Here's how the part is built. I have some questions about the finished solid (model axes, mm). Round coordinates to 2 decimals unless told otherwise and drop trailing zeros. Loops run counter-clockwise (first coordinate to the right, second up) from the corner with the lowest first, then second, coordinate; pieces in that order, holes last. Notation, with made-up numbers: M 89,68.5 L 102,68.5 A15 ccw 102,97.5 Z; hole C 44,-24.5 d9. An arc over 180 degrees is marked long. Use a Markdown table: item, result.
```python
from build123d import *

# Parameters (mm, degrees)
SKETCH_1_W      = 100
SKETCH_1_H      = 160
SKETCH_1_R      = 1.5
SKETCH_1_R_2    = 1.3
SKETCH_1_R_3    = 1.2
SKETCH_1_R_4    = 1.25
SKETCH_1_W_2    = 35
SKETCH_1_H_2    = 12
SKETCH_1_H_3    = 22
EXTRUDE_1_DEPTH = 3
FILLET_1_R      = 10
FILLET_2_R      = 5


with BuildPart() as part:
    # 草图1 → 凸台-拉伸1 (new body)
    with BuildSketch(Plane(origin=(0, 0, 0), x_dir=(1, 0, 0), z_dir=(0, 1, 0))):
        Rectangle(SKETCH_1_W, SKETCH_1_H)
        with Locations(Location((35, 70, 0), (0, 0, 270))):
            Circle(SKETCH_1_R, mode=Mode.SUBTRACT)
        with Locations(Location((-35, 70, 0), (0, 0, 90))):
            Circle(SKETCH_1_R, mode=Mode.SUBTRACT)
        with Locations(Location((-35, -70, 0), (0, 0, 270))):
            Circle(SKETCH_1_R, mode=Mode.SUBTRACT)
        with Locations(Location((35, -70, 0), (0, 0, 90))):
            Circle(SKETCH_1_R, mode=Mode.SUBTRACT)
        with Locations(Location((0, -2, 0), (0, 0, 270))):
            Circle(SKETCH_1_R_2, mode=Mode.SUBTRACT)
        with Locations(Location((13, -15, 0), (0, 0, 270))):
            Circle(SKETCH_1_R_2, mode=Mode.SUBTRACT)
        with Locations(Location((0, -28, 0), (0, 0, 270))):
            Circle(SKETCH_1_R_2, mode=Mode.SUBTRACT)
        with Locations(Location((-13, -15, 0), (0, 0, 270))):
            Circle(SKETCH_1_R_2, mode=Mode.SUBTRACT)
        with Locations(Location((-16, 26, 0), (0, 0, 270))):
            Circle(SKETCH_1_R_3, mode=Mode.SUBTRACT)
        with Locations(Location((42, 26, 0), (0, 0, 270))):
            Circle(SKETCH_1_R_3, mode=Mode.SUBTRACT)
        with Locations(Location((42, 75, 0), (0, 0, 270))):
            Circle(SKETCH_1_R_3, mode=Mode.SUBTRACT)
        with Locations(Location((-16, 75, 0), (0, 0, 270))):
            Circle(SKETCH_1_R_3, mode=Mode.SUBTRACT)
        with Locations(Location((-27.75, -75, 0), (0, 0, 270))):
            Circle(SKETCH_1_R_4, mode=Mode.SUBTRACT)
        with Locations(Location((27.75, -75, 0), (0, 0, 270))):
            Circle(SKETCH_1_R_4, mode=Mode.SUBTRACT)
        with Locations(Location((27.75, -45, 0), (0, 0, 270))):
            Circle(SKETCH_1_R_4, mode=Mode.SUBTRACT)
        with Locations(Location((-27.75, -45, 0), (0, 0, 270))):
            Circle(SKETCH_1_R_4, mode=Mode.SUBTRACT)
        with Locations((0, -62)):
            Rectangle(SKETCH_1_W_2, SKETCH_1_H_2, mode=Mode.SUBTRACT)
        with Locations((13, 50.5)):
            Rectangle(SKETCH_1_W_2, SKETCH_1_H_3, mode=Mode.SUBTRACT)
        with BuildLine():
            Line((-43, -25), (-43, 25))
            ThreePointArc((-43, 25), (-38, 30), (-33, 25))
            Line((-33, 25), (-33, -25))
            ThreePointArc((-33, -25), (-38, -30), (-43, -25))
        make_face(mode=Mode.SUBTRACT)
    extrude(amount=EXTRUDE_1_DEPTH)

    # 圆角1
    fillet_1_edges = [part.edges().sort_by_distance(p)[0] for p in [
        (50, 1.5, 80),
        (-50, 1.5, 80),
        (-50, 1.5, -80),
        (50, 1.5, -80),
    ]]
    fillet(fillet_1_edges, radius=FILLET_1_R)

    # 圆角2
    fillet_2_edges = [part.edges().sort_by_distance(p)[0] for p in [
        (17.5, 1.5, 68),
        (17.5, 1.5, 56),
        (-17.5, 1.5, 56),
        (-17.5, 1.5, 68),
        (30.5, 1.5, -39.5),
        (30.5, 1.5, -61.5),
        (-4.5, 1.5, -61.5),
        (-4.5, 1.5, -39.5),
    ]]
    fillet(fillet_2_edges, radius=FILLET_2_R)


solid = part.part
```
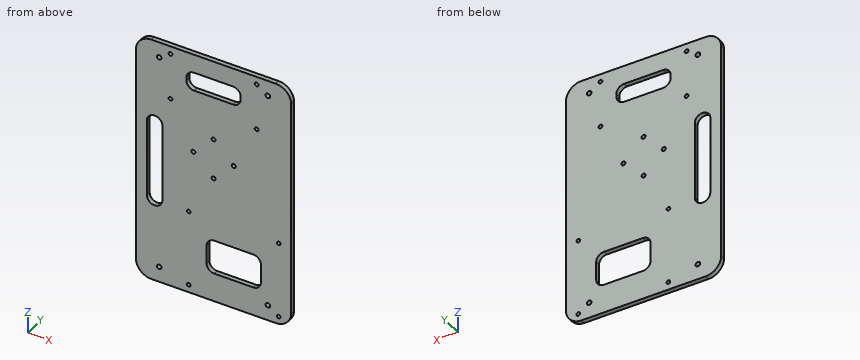
Q1. Will this pin go through, and if not, where does the flat tip stop? P1, Ø4, axis at x = 0, z = 2, coming from the +Y side.
Return value:
| item | result |
|---|---|
| P1 | stops at y = 3 |
Q2. Imagine slicing it at C-C, the plane z = -2. Please give me the cut outline in (x, y), then the cut area to 3 significant figures.
Return value:
| item | result |
|---|---|
| outline | M -50,0 L -43,0 L -43,3 L -50,3 Z; M -33,0 L 50,0 L 50,3 L -33,3 Z |
| area | 270 mm^2 |
Q3. I need wall thicknesses on line 1 (Z direction, x = -28, y = 2.4); line 2 (X direction, y = 1.6, z = -70); line 3 (Z direction, x = 4.5, y = 2.1). Which ranges of each line are inside material? Lowest first, please. Write a range as from..to.
Return value:
| item | result |
|---|---|
| line 1 | z = -80..43.78, 46.22..73.78, 76.22..80 |
| line 2 | x = -50..-36.5, -33.5..33.5, 36.5..50 |
| line 3 | z = -80..-61.5, -39.5..56, 68..80 |
Q4. Imagine slicing it at A-A, the plane z = -41.5. Please give me the cut outline in (x, y).
Return value:
| item | result |
|---|---|
| outline | M -50,0 L -3.5,0 L -3.5,3 L -50,3 Z; M 29.5,0 L 50,0 L 50,3 L 29.5,3 Z |
Q5. Imagine slicing it at B-B, the plane y = 1.7. Give the number of separate pieces and of enclosed holes in the cut face, then the cut area to 3 significant figures.
Return value:
| item | result |
|---|---|
| separate pieces | 1 |
| enclosed holes | 19 |
| area | 14,100 mm^2 |
